from build123d import *

# Parameters (mm, degrees)
SKETCH1_R                = 8
SKETCH1_R_2              = 4
BOSS_EXTRUDE1_DEPTH      = 9
BOSS_EXTRUDE1_2_DEPTH    = 9
SKETCH2_R                = 4
BOSS_EXTRUDE3_DEPTH      = 9
FILLET1_R                = 1
CUT_EXTRUDE1_DEPTH       = 214.789616212
SKETCH4_W                = 9
SKETCH4_H                = 27
BOSS_EXTRUDE4_DEPTH      = 75
BOSS_EXTRUDE5_START      = 9
SKETCH5_R                = 25
SKETCH5_R_2              = 4
BOSS_EXTRUDE5_DEPTH      = 9
BOSS_EXTRUDE6_DEPTH      = 4.5
BOSS_EXTRUDE6_DEPTH_BACK = 4.5
BOSS_EXTRUDE7_DEPTH      = 4.5
BOSS_EXTRUDE7_DEPTH_BACK = 4.5
BOSS_EXTRUDE7_START      = -25
SKETCH9_W                = 9
SKETCH9_H                = 7
SKETCH9_H_2              = 9
CUT_EXTRUDE2_DEPTH       = 217.612557346
CUT_EXTRUDE3_DEPTH       = 216.299790989
CUT_EXTRUDE3_DEPTH_BACK  = 216.299790989
CAVITY1_START            = -66
CAVITY1_OUTLINE_W        = 9
CAVITY1_OUTLINE_H        = 9
CAVITY1_DEPTH            = 26.25
CAVITY1_START_2          = -35.25
CAVITY1_2_OUTLINE_W      = 9
CAVITY1_2_OUTLINE_H      = 9
CAVITY1_2_DEPTH          = 26.25
CAVITY1_START_3          = -56
CAVITY1_3_OUTLINE_W      = 9
CAVITY1_3_OUTLINE_H      = 9
CAVITY1_3_OUTLINE_W_2    = 4.5
CAVITY1_3_DEPTH          = 9
CAVITY1_START_4          = -28
CAVITY1_4_OUTLINE_W      = 9
CAVITY1_4_OUTLINE_H      = 9
CAVITY1_4_OUTLINE_W_2    = 4.5
CAVITY1_4_DEPTH          = 9


# Read off the part's stored shape, not the designer's step: Cavity1
with BuildPart() as part:
    # Sketch1 → Boss-Extrude1 (new body)
    with BuildSketch(Plane.XY):
        with Locations((-125, 0)):
            Circle(SKETCH1_R)
        with Locations((-125, 0)):
            Circle(SKETCH1_R_2, mode=Mode.SUBTRACT)
    extrude(amount=BOSS_EXTRUDE1_DEPTH)



with BuildPart() as body_2:
    # Sketch1 → Boss-Extrude1 2 (new body)
    with BuildSketch(Plane.XY):
        with Locations((125, 0)):
            Circle(SKETCH1_R)
        with Locations((125, 0)):
            Circle(SKETCH1_R_2, mode=Mode.SUBTRACT)
    extrude(amount=BOSS_EXTRUDE1_2_DEPTH)


with BuildPart() as part_1:
    add(part.part)

    add(body_2.part)  # Boss-Extrude3 merges body 2
    # Sketch2 → Boss-Extrude3 (add)
    with BuildSketch(Plane.XY):
        with BuildLine():
            Line((-175, -75), (125, -75))
            ThreePointArc((125, -75), (130.131670325, -43.377223009), (145.000000492, -14.999999344))
            ThreePointArc((145.000000492, -14.999999344), (143.981414944, 16.269784471), (113.235294528, 22.058823748))
            ThreePointArc((113.235294528, 22.058823748), (25.000000075, 0), (-63.235294395, 22.058823677))
            ThreePointArc((-63.235294395, 22.058823677), (-75.420498385, 24.996463372), (-87.499999896, 21.650635154))
            ThreePointArc((-87.499999896, 21.650635154), (-99.999999954, 18.301270189), (-112.500000024, 21.650635108))
            ThreePointArc((-112.500000024, 21.650635108), (-124.99999995, 25), (-137.49999989, 21.650635158))
            ThreePointArc((-137.49999989, 21.650635158), (-149.999999954, 18.301270189), (-162.50000003, 21.650635112))
            ThreePointArc((-162.50000003, 21.650635112), (-193.705072901, 16.586749162), (-195.000000551, -14.999999265))
            ThreePointArc((-195.000000551, -14.999999265), (-180.13167034, -43.377222962), (-175, -75))
        make_face()
        with Locations((125, 0)):
            Circle(SKETCH2_R, mode=Mode.SUBTRACT)
        with Locations((-175, 0)):
            Circle(SKETCH2_R, mode=Mode.SUBTRACT)
        with Locations((-125, 0)):
            Circle(SKETCH2_R, mode=Mode.SUBTRACT)
        with Locations((-75, 0)):
            Circle(SKETCH2_R, mode=Mode.SUBTRACT)
    extrude(amount=BOSS_EXTRUDE3_DEPTH)

    # Fillet1
    fillet1_edges = [part_1.edges().sort_by_distance(p)[0] for p in [
        (-175, -75, 4.5),
        (125, -75, 4.5),
    ]]
    fillet(fillet1_edges, radius=FILLET1_R)

    # Sketch3 → Cut-Extrude1 (cut, through all)
    with BuildSketch(Plane.XY):
        Polygon((25, 0), (25, -75), (150, -75), (150, 25), (25, 25), align=None)
    extrude(amount=CUT_EXTRUDE1_DEPTH, mode=Mode.SUBTRACT)

    # Sketch4 → Boss-Extrude4 (add)
    with BuildSketch(Plane.XZ.offset(75)):
        with Locations((25, -4.5)):
            Rectangle(SKETCH4_W, SKETCH4_H)
    extrude(amount=-BOSS_EXTRUDE4_DEPTH)

    # Sketch5 → Boss-Extrude5 (add)
    # profile 1 of 4: a face of its own
    with BuildSketch(Plane(origin=(0, 0, -18), x_dir=(-1, 0, 0), z_dir=(0, 0, -1)).offset(BOSS_EXTRUDE5_START)):
        with BuildLine():
            ThreePointArc((-145.000000304, -14.999999594), (-130.131670275, -43.377223158), (-125, -75))
            Line((-125, -75), (-29.5, -75))
            Line((-29.5, -75), (-29.5, 0))
            Line((-29.5, 0), (-100, 0))
            ThreePointArc((-100, 0), (-117.09430609, -23.717082532), (-145.000000304, -14.999999594))
        make_face()
    # profile 2 of 4: a face of its own
    with BuildSketch(Plane(origin=(0, 0, -18), x_dir=(-1, 0, 0), z_dir=(0, 0, -1)).offset(BOSS_EXTRUDE5_START)):
        with Locations((-125, 0)):
            Circle(SKETCH5_R)
        with Locations((-125, 0)):
            Circle(SKETCH5_R_2, mode=Mode.SUBTRACT)
    # profile 3 of 4: a face of its own
    with BuildSketch(Plane(origin=(0, 0, -18), x_dir=(-1, 0, 0), z_dir=(0, 0, -1)).offset(BOSS_EXTRUDE5_START)):
        Polygon((-29.5, 0), (-29.5, -75), (-20.5, -75), (-20.5, 0), (-25, 0), align=None)
    # profile 4 of 4: a face of its own
    with BuildSketch(Plane(origin=(0, 0, -18), x_dir=(-1, 0, 0), z_dir=(0, 0, -1)).offset(BOSS_EXTRUDE5_START)):
        with BuildLine():
            Line((-100, 0), (-29.5, 0))
            Line((-29.5, 0), (-25, 0))
            ThreePointArc((-25, 0), (-70.475429529, 5.598281181), (-113.235293817, 22.058823369))
            ThreePointArc((-113.235293817, 22.058823369), (-103.56267677, 12.86239374), (-100, 0))
        make_face()
    extrude(amount=-BOSS_EXTRUDE5_DEPTH)

    # Sketch7 → Boss-Extrude6 (add, two sides: drawn at the far end of the back side and taken through both)
    with BuildSketch(Plane(origin=(0, -25, 0), x_dir=(1, 0, 0), z_dir=(0, 1, 0)).offset(-BOSS_EXTRUDE6_DEPTH_BACK)):
        with BuildLine():
            Line((56.5, 18), (29.5, 18))
            Line((29.5, 18), (29.5, -9))
            ThreePointArc((29.5, -9), (48.591883092, -1.091883092), (56.5, 18))
        make_face()
        with BuildLine():
            Line((-6.5, 0), (20.5, 0))
            Line((20.5, 0), (20.5, 27))
            ThreePointArc((20.5, 27), (1.408116908, 19.091883092), (-6.5, 0))
        make_face()
    extrude(amount=BOSS_EXTRUDE6_DEPTH + BOSS_EXTRUDE6_DEPTH_BACK)

    # Sketch7<3> → Boss-Extrude7 (add, two sides: drawn at the far end of the back side and taken through both)
    with BuildSketch(Plane(origin=(0, -25, 0), x_dir=(1, 0, 0), z_dir=(0, 1, 0)).offset(BOSS_EXTRUDE7_START - BOSS_EXTRUDE7_DEPTH_BACK)):
        with BuildLine():
            Line((56.5, 18), (29.5, 18))
            Line((29.5, 18), (29.5, -9))
            ThreePointArc((29.5, -9), (48.591883092, -1.091883092), (56.5, 18))
        make_face()
        with BuildLine():
            Line((-6.5, 0), (20.5, 0))
            Line((20.5, 0), (20.5, 27))
            ThreePointArc((20.5, 27), (1.408116908, 19.091883092), (-6.5, 0))
        make_face()
    extrude(amount=BOSS_EXTRUDE7_DEPTH + BOSS_EXTRUDE7_DEPTH_BACK)

    # Sketch9 → Cut-Extrude2 (cut, through all)
    with BuildSketch(Plane.XY.offset(9)):
        with Locations((-160.208548161, -53.5)):
            Rectangle(SKETCH9_W, SKETCH9_H)
        with Locations((-160.208548161, -70.5)):
            Rectangle(SKETCH9_W, SKETCH9_H_2)
        with Locations((-25.351798772, -53.5)):
            Rectangle(SKETCH9_W, SKETCH9_H)
        with Locations((-25.351798772, -70.5)):
            Rectangle(SKETCH9_W, SKETCH9_H_2)
        with Locations((109.504950616, -53.5)):
            Rectangle(SKETCH9_W, SKETCH9_H)
        with Locations((109.504950616, -70.5)):
            Rectangle(SKETCH9_W, SKETCH9_H_2)
    extrude(amount=-CUT_EXTRUDE2_DEPTH, mode=Mode.SUBTRACT)

    # Sketch10 → Cut-Extrude3 (cut, two sides: drawn at the far end of the back side and taken through both)
    with BuildSketch(Plane(origin=(0, 0, 0), x_dir=(1, 0, 0), z_dir=(0, 1, 0)).offset(-CUT_EXTRUDE3_DEPTH_BACK)):
        Polygon((-200, 27), (-200, 0), (25, 0), (25, -9), (150, -9), (150, 18), (20.5, 18), (20.5, 27), align=None)
    extrude(amount=CUT_EXTRUDE3_DEPTH + CUT_EXTRUDE3_DEPTH_BACK, mode=Mode.SUBTRACT)


with BuildPart() as cut_extrude3_kept_piece:
    # of the separate pieces the step leaves, the one the design keeps (cut_extrude3_pieces_kept)
    add(part_1.part.solids().sort_by_distance((20.5, 0, -27))[0])

    # Cavity1 outline → Cavity1 (cut)
    with BuildSketch(Plane(origin=(0, 0, 0), x_dir=(1, 0, 0), z_dir=(0, 1, 0)).offset(CAVITY1_START)):
        with Locations((25, 22.5)):
            Rectangle(CAVITY1_OUTLINE_W, CAVITY1_OUTLINE_H)
    extrude(amount=CAVITY1_DEPTH, mode=Mode.SUBTRACT)

    # Cavity1 2 outline → Cavity1 2 (cut)
    with BuildSketch(Plane(origin=(0, 0, 0), x_dir=(1, 0, 0), z_dir=(0, 1, 0)).offset(CAVITY1_START_2)):
        with Locations((25, 22.5)):
            Rectangle(CAVITY1_2_OUTLINE_W, CAVITY1_2_OUTLINE_H)
    extrude(amount=CAVITY1_2_DEPTH, mode=Mode.SUBTRACT)

    # Cavity1 3 outline → Cavity1 3 (cut)
    with BuildSketch(Plane(origin=(0, 0, 0), x_dir=(1, 0, 0), z_dir=(0, 1, 0)).offset(CAVITY1_START_3)):
        with Locations((52, 22.5)):
            Rectangle(CAVITY1_3_OUTLINE_W, CAVITY1_3_OUTLINE_H)
        with Locations((40.75, 22.5)):
            Rectangle(CAVITY1_3_OUTLINE_W_2, CAVITY1_3_OUTLINE_H)
    extrude(amount=CAVITY1_3_DEPTH, mode=Mode.SUBTRACT)

    # Cavity1 4 outline → Cavity1 4 (cut)
    with BuildSketch(Plane(origin=(0, 0, 0), x_dir=(1, 0, 0), z_dir=(0, 1, 0)).offset(CAVITY1_START_4)):
        with Locations((52, 22.5)):
            Rectangle(CAVITY1_4_OUTLINE_W, CAVITY1_4_OUTLINE_H)
        with Locations((40.75, 22.5)):
            Rectangle(CAVITY1_4_OUTLINE_W_2, CAVITY1_4_OUTLINE_H)
    extrude(amount=CAVITY1_4_DEPTH, mode=Mode.SUBTRACT)


solid = cut_extrude3_kept_piece.part
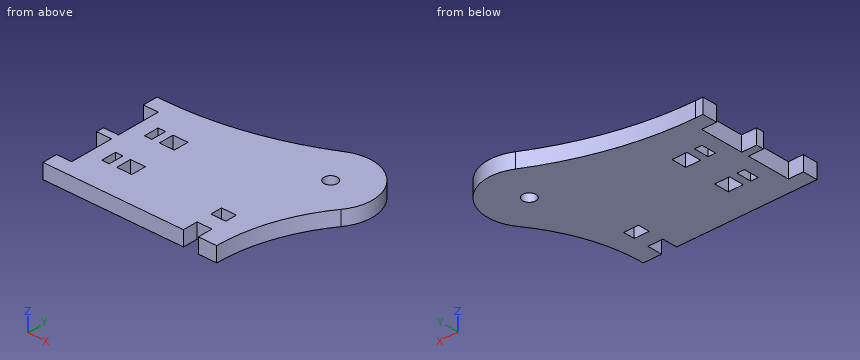
Input: part model. Units: mm. Frame: model coordinates. Round coordinates to 2 decimals unless told otherwise and drop trailing zeros. Loops run counter-clockwise (first coordinate to the right, second up) from the corner with the lowest first, then second, coordinate; pieces in that order, holes last. Notation, with made-up numbers: (-25.75, 41) -> (33.25, 41) arc R36 ccw to (33.25, 79) -> close; hole circle Ø10 at (77.25, -40). An arc over 180 degrees is marked (long way). Answer as a JSON object with one key per item and string values. Group by question number.
1) Section query C-C on x = 97.5. Output: boundary loops of the cut face in (y, z), plus the area to 3 significant figures.
2) Ray query, L1, parallel to Y at x = 50.5, z = -19; L2, parallel to Y at x = 49, z = -18.75; L3, parallel to X at y = -2, z = -22.25. Return the intervals inside material, ascending.
3) Section query A-A on y = -25.5. Output: boundary loops of the cut face in (x, z), plus the area to 3 significant figures.
4) Pin query (flat end, axial travel): pin 1 (4.5 mm diameter, centred on x = 26.5, z = -24.5, fed in from +Y); pin 2 (2 mm diameter, centred on x = 83.5, z = -24.5, fed in from +Y); pin 3 (3.5 mm diameter, centred on x = 41.5, z = -22, fed in from +Y); pin 4 (7 mm diameter, centred on x = 125, y = 0, fed in from +Z). Return the tip coordinate at first contact, or that it passes through.
5) Section query B-B on z = -25.25. State how many separate pieces and enclosed holes the cut face has, plus the area to 3 significant figures.
Reply:
{
 "1": {"outline": "(-75, -27) -> (14.58, -27) -> (14.58, -18) -> (-75, -18) -> close", "area": "806 mm2"},
 "2": {"L1": "y = -75 to -56, -47 to -28, -19 to 1.74", "L2": "y = -75 to -56, -47 to -28, -19 to 1.54", "L3": "x = 20.5 to 121.54, 128.46 to 149.92"},
 "3": {"outline": "(29.5, -27) -> (38.5, -27) -> (38.5, -18) -> (29.5, -18) -> close; (43, -27) -> (47.5, -27) -> (47.5, -18) -> (43, -18) -> close; (56.5, -27) -> (138.11, -27) -> (138.11, -18) -> (56.5, -18) -> close", "area": "856 mm2"},
 "4": {"pin 1": "stops at y = 0.04", "pin 2": "stops at y = 9.69", "pin 3": "stops at y = 0.89", "pin 4": "passes through"},
 "5": {"separate pieces": "1", "enclosed holes": "6", "area": "9,070 mm2"}
}
